from build123d import *

# Parameters (mm, degrees)
F0_R     = 31
F1_DEPTH = 44
F2_R     = 31
F2_R_2   = 20
F3_DEPTH = 32
F5_DEPTH = 25
F7_DEPTH = 16


with BuildPart() as f1:
    # F0 (on Right) → F1 (new body)
    with BuildSketch(Plane.YZ):
        Circle(F0_R)
    extrude(amount=F1_DEPTH)

    # F2 (on face) → F3 (cut)
    with BuildSketch(Plane.YZ.offset(44)):
        Circle(F2_R)
        Circle(F2_R_2, mode=Mode.SUBTRACT)
    extrude(amount=-F3_DEPTH, mode=Mode.SUBTRACT)

    # F4 (on face) → F5 (cut)
    with BuildSketch(Plane.YZ.offset(12)):
        with BuildLine():
            ThreePointArc((6, 30.4138126515), (0, 31), (-6, 30.4138126515))
            Line((-6, 30.4138126515), (-6, 19.0787840283))
            ThreePointArc((-6, 19.0787840283), (0, 20), (6, 19.0787840283))
            Line((6, 19.0787840283), (6, 30.4138126515))
        make_face()
        with BuildLine():
            Line((-6, -19.0787840283), (-6, -30.4138126515))
            ThreePointArc((-6, -30.4138126515), (0, -31), (6, -30.4138126515))
            Line((6, -30.4138126515), (6, -19.0787840283))
            ThreePointArc((6, -19.0787840283), (0, -20), (-6, -19.0787840283))
        make_face()
    extrude(amount=-F5_DEPTH, mode=Mode.SUBTRACT)

    # F6 (on face) → F7 (cut)
    with BuildSketch(Plane.YZ.offset(44)):
        with BuildLine():
            Line((-19.7737199333, -3), (-6.3245553203, -3))
            ThreePointArc((-6.3245553203, -3), (0, -7), (6.3245553203, -3))
            Line((6.3245553203, -3), (19.7737199333, -3))
            ThreePointArc((19.7737199333, -3), (19.9433497521, -1.5042608375), (20, 0))
            ThreePointArc((20, 0), (19.9433497521, 1.5042608375), (19.7737199333, 3))
            Line((19.7737199333, 3), (6.3245553203, 3))
            ThreePointArc((6.3245553203, 3), (0, 7), (-6.3245553203, 3))
            Line((-6.3245553203, 3), (-19.7737199333, 3))
            ThreePointArc((-19.7737199333, 3), (-20, 0), (-19.7737199333, -3))
        make_face()
    extrude(amount=-F7_DEPTH, mode=Mode.SUBTRACT)


solid = f1.part
Design review of the part built by this model. Coordinates are the model's own, in mm. A direction names the side the tool comes from. Give positions to 0.01 mm unless a question says otherwise; leave off trailing zeros. Write each loop counter-clockwise with the first axis right and the second up, starting at its lowest first coordinate (ties: lowest second). Pieces come first, ordered by that corner, then holes. Notation, with made-up numbers: M 55.25,71.25 L 89.25,71.25 A20 cw 89.25,76.25 Z; hole C -29.75,38.25 d3. An arc over 180 degrees is marked long. Return JSON: item names as keys, results as strings. Group by question number.
Item 1: Tool access review of faces 4 (the flat face through (6, -6, -25)), 5 (the cylindrical face through (36, 0, 7)), 6 (the flat face through (6, -6, 25)), 7 (the flat face through (12, -21, 0)), 8 (the flat face through (36, -13, -3)): name each direction out of +Z, -Z, +X, -X, +Y, -Y from which nothing blocks a thin tool from reaching the whole face with its end or side.
Item 2: Clearance check with flat-ended pins moving along their axes: pin 1 Ø9 at (x, z) = (7, 23) entering from -Y; pin 2 Ø8 at (x, y) = (10.5, 19) entering from -Z; pin 3 Ø15 at (x, y) = (34, 13) entering from -Z. State where each tip first meets the part, or that it passes through.
Item 3: The part is to be moulded in two halves that separate along Z. For faces 1 (the flat face through (36, 13, 3)), 2 (the flat face through (12, 21, 0)), 3 (the cylindrical face through (5.916, 30.994, -0.597)), say which applies: pulls with the +Z half, pulls with the -Z half, needs draft (parallel to the pull), parting line crosses it, or undercut.
Item 4: Take a section at C-C (y = 0). Give the boundary of the cut face in (x, z), plus the area to 3 significant figures.
Item 5: Take a section at D-D (z = 23). Give the boundary of the cut face in (x, y).
Item 6: Take a section at B-B (z = 0). Give the boundary of the cut face in (x, y), plus the area to 3 significant figures.
Item 7: Wall thickness on line 1 along X through (y, z) = (18, -11.5); line 2 along Y through (x, z) = (14, 0.5); line 3 along Z through (x, y) = (29, 8): over which ranges is each line inside the solid? List them lowest first.
Item 8: Take a section at A-A (x = 39). Give the boundary of the cut face in (y, z).
Return value:
{
 "1": {"face 4": "-Z, +X, -X", "face 5": "+X", "face 6": "+Z, +X, -X", "face 7": "+X, -Y", "face 8": "+X, +Y, -Y"},
 "2": {"pin 1": "stops at y = -24.87", "pin 2": "stops at z = -27.13", "pin 3": "stops at z = -19.23"},
 "3": {"face 1": "undercut", "face 2": "needs draft", "face 3": "parting line crosses it"},
 "4": {"outline": "M 0,-20 L 44,-20 L 44,-7 L 28,-7 L 28,7 L 44,7 L 44,20 L 0,20 Z", "area": "1,540 mm2"},
 "5": {"outline": "M 0,-20.78 L 12,-20.78 L 12,-6 L 0,-6 Z; M 0,6 L 12,6 L 12,20.78 L 0,20.78 Z"},
 "6": {"outline": "M 0,-31 L 12,-31 L 12,-20 L 28,-20 L 28,20 L 12,20 L 12,31 L 0,31 Z", "area": "1,380 mm2"},
 "7": {"line 1": "x = 0 to 12", "line 2": "y = -19.99 to 19.99", "line 3": "z = -18.33 to -3, 3 to 18.33"},
 "8": {"outline": "M -19.77,-3 A20 ccw 19.77,-3 L 6.32,-3 A7 cw -6.32,-3 Z; M -19.77,3 L -6.32,3 A7 cw 6.32,3 L 19.77,3 A20 ccw Z"}
}
